Work out the finished part from the listing and answer in its coordinate system (mm). Face numbers are marked on the shaded views. Round coordinates to 2 decimals unless told otherwise and drop trailing zeros. Loops run counter-clockwise (first coordinate to the right, second up) from the corner with the lowest first, then second, coordinate; pieces in that order, holes last. Notation, with made-up numbers: (70, 15) - (123, 15) arc R21 ccw to (123, 44) - close; hole circle Ø4 at (51.25, 73.5). An arc over 180 degrees is marked (long way). Return JSON: item names as keys, results as strings.
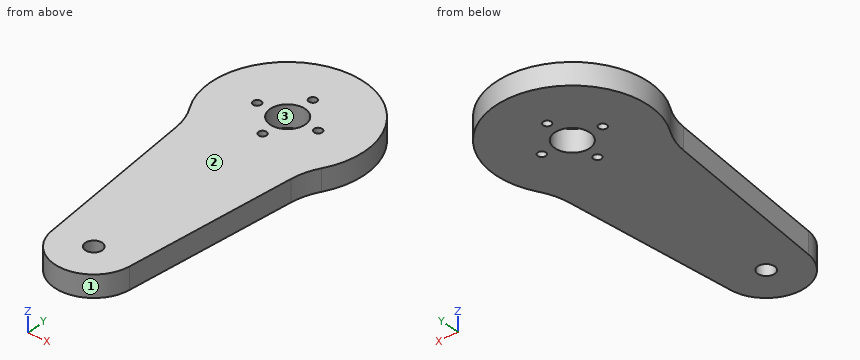
from build123d import *

# Parameters (mm, degrees)
ESQUISSE1_R        = 1.925
ESQUISSE1_R_2      = 0.925
ESQUISSE1_R_3      = 4
BOSS_EXTRU_1_DEPTH = 5


with BuildPart() as part:
    # Esquisse1 → Boss.-Extru.1 (new body)
    with BuildSketch(Plane.XY):
        with BuildLine():
            Line((8.950697062, -54.94075613), (13.146568064, -15.019708545))
            ThreePointArc((13.146568064, -15.019708545), (13.822417384, -11.87955399), (15.151330627, -8.955287839))
            ThreePointArc((15.151330627, -8.955287839), (0, 17.600000001), (-15.151330627, -8.955287839))
            ThreePointArc((-15.151330627, -8.955287839), (-13.822417384, -11.87955399), (-13.146568064, -15.019708545))
            Line((-13.146568064, -15.019708545), (-8.950697062, -54.94075613))
            ThreePointArc((-8.950697062, -54.94075613), (0, -63), (8.950697062, -54.94075613))
        make_face()
        with Locations((0, -54)):
            Circle(ESQUISSE1_R, mode=Mode.SUBTRACT)
        with Locations((7, 0)):
            Circle(ESQUISSE1_R_2, mode=Mode.SUBTRACT)
        with Locations((0, -7)):
            Circle(ESQUISSE1_R_2, mode=Mode.SUBTRACT)
        with Locations((0, 7)):
            Circle(ESQUISSE1_R_2, mode=Mode.SUBTRACT)
        with Locations((-7, 0)):
            Circle(ESQUISSE1_R_2, mode=Mode.SUBTRACT)
        Circle(ESQUISSE1_R_3, mode=Mode.SUBTRACT)
    extrude(amount=BOSS_EXTRU_1_DEPTH)


solid = part.part
1) Determine the mould class of the marked faces 1, 2 and 3 for opening direction Y: pulls with the +Y half, pulls with the -Y half, needs draft (parallel to the pull), parting line crosses it, or undercut.
Verdict:
{"face 1": "pulls with the -Y half", "face 2": "needs draft", "face 3": "undercut"}
2) Section C-C (z = 2.6) is taken. Give the vertices of the cut face in (x, y) (3 decimals).
Verdict:
{"outline": "(-15.151, -8.955) arc R15 cw to (-13.147, -15.02) - (-8.951, -54.941) arc R9 ccw to (8.951, -54.941) - (13.147, -15.02) arc R15 cw to (15.151, -8.955) arc R17.6 ccw (long way) to start; hole circle Ø1.85 at (-7, 0); hole circle Ø8 at (0, 0); hole circle Ø3.85 at (0, -54); hole circle Ø1.85 at (0, -7); hole circle Ø1.85 at (0, 7); hole circle Ø1.85 at (7, 0)"}
3) Section D-D (x = -7) is taken. Give the vertices of the cut face in (y, z) (3 decimals), and give its area (3 significant figures).
Verdict:
{"outline": "(-59.657, 0) - (-0.925, 0) - (-0.925, 5) - (-59.657, 5) - close; (0.925, 0) - (16.148, 0) - (16.148, 5) - (0.925, 5) - close", "area": "370 mm2"}
4) Find the intervals of material crossed by L1, parallel to Y at x = 1.5, z = 1; L2, parallel to X at y = 1.5, z = 2.9; L3, parallel to Y at x = -15, z = 2.7, in increasing order.
Verdict:
{"L1": "y = -62.87 to -55.21, -52.79 to -3.71, 3.71 to 17.54", "L2": "x = -17.54 to -3.71, 3.71 to 17.54", "L3": "y = -9.22 to 9.21"}
5) Section A-A (y = 0) is taken. Give the vertices of the cut face in (x, z) (3 decimals), and give its area (4 significant figures).
Verdict:
{"outline": "(-17.6, 0) - (-7.925, 0) - (-7.925, 5) - (-17.6, 5) - close; (-6.075, 0) - (-4, 0) - (-4, 5) - (-6.075, 5) - close; (4, 0) - (6.075, 0) - (6.075, 5) - (4, 5) - close; (7.925, 0) - (17.6, 0) - (17.6, 5) - (7.925, 5) - close", "area": "117.5 mm2"}
6) Section B-B (x = 0) is taken. Give the vertices of the cut face in (y, z) (3 decimals), and give its area (3 significant figures).
Verdict:
{"outline": "(-63, 0) - (-55.925, 0) - (-55.925, 5) - (-63, 5) - close; (-52.075, 0) - (-7.925, 0) - (-7.925, 5) - (-52.075, 5) - close; (-6.075, 0) - (-4, 0) - (-4, 5) - (-6.075, 5) - close; (4, 0) - (6.075, 0) - (6.075, 5) - (4, 5) - close; (7.925, 0) - (17.6, 0) - (17.6, 5) - (7.925, 5) - close", "area": "325 mm2"}
7) Flat-ended cylindrical pins translate along their axes: pin 1 (10.5 mm diameter, centred on x = 0, y = 0, fed in from +Z); pin 2 (1.5 mm diameter, centred on x = 2, z = 0.5, fed in from -Y); pin 3 (3 mm diameter, centred on y = -21.5, z = 1, fed in from +X); pin 4 (1.5 mm diameter, centred on y = -7, z = 4, fed in from -X). Find the tip coordinate at first contact, or state that the pin passes through.
Verdict:
{"pin 1": "stops at z = 5", "pin 2": "stops at y = -62.91", "pin 3": "stops at x = 12.62", "pin 4": "stops at x = -16.45"}
